```python
from build123d import *

# Parameters (mm, degrees)
F1_DEPTH = 9.525
F2_W     = 50.8
F2_H     = 76.2
F3_DEPTH = 53.975
F5_DEPTH = 50.8
F6_R     = 19.05
F7_DEPTH = 76.2


with BuildPart() as f1:
    # F0 (on Top) → F1 (new body)
    with BuildSketch(Plane.XY):
        Polygon((0, 38.1), (-38.1, 38.1), (-38.1, 0), (-38.1, -38.1), (0, -38.1), (38.1, -38.1), (38.1, 0), (38.1, 38.1), align=None)
    extrude(amount=F1_DEPTH)

    # F2 (on face) → F3 (join)
    with BuildSketch(Plane.XY.offset(9.525)):
        Rectangle(F2_W, F2_H)
    extrude(amount=F3_DEPTH)

    # F4 (on face) → F5 (cut)
    with BuildSketch(Plane(origin=(-25.4, 0, 0), x_dir=(0, -1, 0), z_dir=(-1, 0, 0))):
        Polygon((-38.1, 63.5), (-38.1, 38.1), (-12.7, 63.5), align=None)
        Polygon((38.1, 63.5), (0, 63.5), (38.1, 25.4), align=None)
    extrude(amount=-F5_DEPTH, mode=Mode.SUBTRACT)

    # F6 (on face) → F7 (cut)
    with BuildSketch(Plane(origin=(0, -31.75, 31.75), x_dir=(1, 0, 0), z_dir=(0, -0.707107, 0.707107))):
        with Locations((0, 19.501281)):
            Circle(F6_R)
    extrude(amount=-F7_DEPTH, mode=Mode.SUBTRACT)


solid = f1.part
```
Here's how the part is built. I have some questions about the finished solid (model axes, mm). A direction names the side the tool comes from. Coordinates: 2 decimals unless noted, no trailing zeros. Order: outer loops, then holes, each group sorted by start corner. A loop starts at its lowest first (then second) coordinate and runs counter-clockwise, first axis right, second up.
Item 1: I need wall thicknesses on probe 1 along X at (y, z) = (-30.5, 12); probe 2 along Z at (x, y) = (-35, 14) (3 decimals); probe 3 along Y at (x, z) = (1.5, 17). Which ranges of each line are inside material? Lowest first, please.
Response values:
probe 1: x = -25.4 to 25.4
probe 2: z = 0 to 9.525
probe 3: y = -38.1 to -16.28, 37.44 to 38.1
Item 2: If we section it at C-C, the plane x = -1: List the corners of the cut face in (y, z) for me, then the cut area to 3 significant figures.
Response values:
outline: (-38.1, 0) - (0.68, 0) - (-31.41, 32.09) - (-38.1, 25.4) - close; (-4.51, 58.99) - (38.1, 16.38) - (38.1, 38.1) - (12.7, 63.5) - (0, 63.5) - close
area: 1,470 mm2
Item 3: Which directions (+Z, -Z, +X, -X, +Y, -Y) give clear straight access to the entire face, cutting with the end or side of a thin tool? Please do faces 4 (the face through (-1, -38.1, 13)), 5 (the face through (-25.4, -1, 30)), 6 (the face through (25.4, -1, 30)).
Response values:
face 4: +Z, -Z, +X, -X, -Y
face 5: +Z, -X, +Y, -Y
face 6: +Z, +X, +Y, -Y
Item 4: If we section it at B-B, the plane x = -23: List the corners of the cut face in (y, z) for me.
Response values:
outline: (-38.1, 0) - (38.1, 0) - (38.1, 38.1) - (12.7, 63.5) - (0, 63.5) - (-38.1, 25.4) - close
Item 5: If we section it at A-A, the plane x = 11: List the corners of the cut face in (y, z) for me.
Response values:
outline: (-38.1, 0) - (5.58, 0) - (-28.96, 34.54) - (-38.1, 25.4) - close; (-6.96, 56.54) - (38.1, 11.47) - (38.1, 38.1) - (12.7, 63.5) - (0, 63.5) - close
Item 6: If we section it at D-D, the plane x = 31.5: List the corners of the cut face in (y, z) for me (3 decimals).
Response values:
outline: (-38.1, 0) - (38.1, 0) - (38.1, 9.525) - (-38.1, 9.525) - close
Item 7: I'm going to push flat-ended pins straight in: pin 1 Ø8 at (x, z) = (0, 39.5) entering from -Y; pin 2 Ø4 at (y, z) = (21, 23) entering from +X; pin 3 Ø14 at (x, y) = (31.5, 0.5) entering from +Z; pin 4 Ø6 at (y, z) = (8, 36) entering from -X. Where does each tip first touch, or does it pass through?
Response values:
pin 1: stops at y = 11.02
pin 2: stops at x = 25.4
pin 3: stops at z = 63.5
pin 4: stops at x = -25.4
Item 8: Thinking about a two-plate mould opening in Z: for faces 1 (the face through (-2.48, 14.795, 39.495)), 2 (the face through (-1, -8, 0)), 3 (the face through (32, 1, 9.525)), which applies, pulls with the +Z half, pulls with the -Z half, needs draft (parallel to the pull), parting line crosses it, or undercut?
Response values:
face 1: undercut
face 2: pulls with the -Z half
face 3: pulls with the +Z half
